from build123d import *

# Parameters (mm, degrees)
SKETCH1_R                = 67.8
SKETCH1_R_2              = 50
BOSS_EXTRUDE1_DEPTH      = 10
BOSS_EXTRUDE4_DEPTH      = 10
BOSS_EXTRUDE4_DEPTH_BACK = 10
SKETCH2_R                = 25
SKETCH2_R_2              = 67.8
CUT_EXTRUDE1_START       = -20
CUT_EXTRUDE1_DEPTH       = 20


# Read off the part's stored shape, not the designer's step: Cut-Extrude1
with BuildPart() as part:
    # Sketch1 → Boss-Extrude1 (new body)
    with BuildSketch(Plane(origin=(0, 0, 0), x_dir=(1, 0, 0), z_dir=(0, 1, 0))):
        with Locations(Location((0, 0, 0), (0, 0, 270))):
            Circle(SKETCH1_R)
        with Locations(Location((0, 0, 0), (0, 0, 270))):
            Circle(SKETCH1_R_2, mode=Mode.SUBTRACT)
    extrude(amount=BOSS_EXTRUDE1_DEPTH)

    # Sketch2 → Boss-Extrude4 (add, two sides: drawn at the far end of the back side and taken through both)
    with BuildSketch(Plane(origin=(0, 10, 0), x_dir=(1, 0, 0), z_dir=(0, 1, 0)).offset(-BOSS_EXTRUDE4_DEPTH_BACK)):
        with BuildLine():
            ThreePointArc((150, -40), (190, 0), (150, 40))
            ThreePointArc((150, 40), (134.692662705, 36.9551813), (121.715728753, 28.284271247))
            add(Edge.make_bspline(
                [(53.033008589, 53.033008589), (65.214190565, 40.851826613), (81.157405982, 26.386889755), (111.148754798, 17.717297293), (121.715728753, 28.284271247)],
                knots=[0, 0, 0, 0, 0.557862637, 1, 1, 1, 1], degree=3))
            ThreePointArc((53.033008589, 53.033008589), (0, 75), (-53.033008589, 53.033008589))
            add(Edge.make_bspline(
                [(-53.033008589, 53.033008589), (-65.214190565, 40.851826613), (-81.157405982, 26.386889755), (-111.148754798, 17.717297293), (-121.715728753, 28.284271247)],
                knots=[0, 0, 0, 0, 0.557862637, 1, 1, 1, 1], degree=3))
            ThreePointArc((-121.715728753, 28.284271247), (-134.692662705, 36.9551813), (-150, 40))
            ThreePointArc((-150, 40), (-190, 0), (-150, -40))
            ThreePointArc((-150, -40), (-134.692662705, -36.9551813), (-121.715728753, -28.284271247))
            add(Edge.make_bspline(
                [(-53.033008589, -53.033008589), (-65.214190565, -40.851826613), (-81.157405982, -26.386889755), (-111.148754798, -17.717297293), (-121.715728753, -28.284271247)],
                knots=[0, 0, 0, 0, 0.557862637, 1, 1, 1, 1], degree=3))
            ThreePointArc((-53.033008589, -53.033008589), (0, -75), (53.033008589, -53.033008589))
            add(Edge.make_bspline(
                [(53.033008589, -53.033008589), (65.214190565, -40.851826613), (81.157405982, -26.386889755), (111.148754798, -17.717297293), (121.715728753, -28.284271247)],
                knots=[0, 0, 0, 0, 0.557862637, 1, 1, 1, 1], degree=3))
            ThreePointArc((121.715728753, -28.284271247), (134.692662705, -36.9551813), (150, -40))
        make_face()
        with Locations(Location((-150, 0, 0), (0, 0, 270))):
            Circle(SKETCH2_R, mode=Mode.SUBTRACT)
        with Locations(Location((0, 0, 0), (0, 0, 270))):
            Circle(SKETCH2_R_2, mode=Mode.SUBTRACT)
        with Locations(Location((150, 0, 0), (0, 0, 270))):
            Circle(SKETCH2_R, mode=Mode.SUBTRACT)
    extrude(amount=BOSS_EXTRUDE4_DEPTH + BOSS_EXTRUDE4_DEPTH_BACK)

    # Cut-Extrude1 outline → Cut-Extrude1 (cut)
    with BuildSketch(Plane(origin=(0, 20, 0), x_dir=(1, 0, 0), z_dir=(0, 1, 0)).offset(CUT_EXTRUDE1_START)):
        with BuildLine():
            ThreePointArc((188.729833462, -10), (190, 0), (188.729833462, 10))
            Line((188.729833462, 10), (172.912878475, 10))
            ThreePointArc((172.912878475, 10), (175, 0), (172.912878475, -10))
            Line((172.912878475, -10), (188.729833462, -10))
        make_face()
        with BuildLine():
            ThreePointArc((-172.912878475, -10), (-175, 0), (-172.912878475, 10))
            Line((-172.912878475, 10), (-188.729833462, 10))
            ThreePointArc((-188.729833462, 10), (-190, 0), (-188.729833462, -10))
            Line((-188.729833462, -10), (-172.912878475, -10))
        make_face()
    extrude(amount=CUT_EXTRUDE1_DEPTH, mode=Mode.SUBTRACT)


solid = part.part
The model under review builds one solid part; all positions refer to its coordinate system, in mm. A direction names the side the tool comes from. Coordinates: 2 decimals unless noted, no trailing zeros. Loops run counter-clockwise (first coordinate to the right, second up) from the corner with the lowest first, then second, coordinate; pieces in that order, holes last.
(1) Tool access review of faces 5 (the cylindrical face through (15.02, 4.93, 47.69)), 6 (the flat face through (-50, 10, -5)), 7 (the flat face through (-181, 10, -10)), 8 (the flat face through (181, 10, 10)): name each direction out of +Z, -Z, +X, -X, +Y, -Y from which nothing blocks a thin tool from reaching the whole face with its end or side.
Determined:
face 5: +Y, -Y
face 6: +Y
face 7: -X, +Y, -Y
face 8: +X, +Y, -Y
(2) Consider section D-D, the plane z = 56.5. Give the boundary of the cut face in (x, y), plus the area to 3 significant figures.
Determined:
outline: (-49.32, 0) - (49.32, 0) - (49.32, 20) - (37.48, 20) - (37.48, 10) - (-37.48, 10) - (-37.48, 20) - (-49.32, 20) - close
area: 1,220 mm2
(3) Draft analysis for pull direction Z (two halves, no side actions). For faces 1 (the flat face through (13, 20, -67)), 2 (the cylindrical face through (-0.825, 9.86, 74.995)), 3 (the cylindrical face through (125.02, 9.86, -0.96)), 4 (the cylindrical face through (0.825, 9.86, -74.995)), state which applies: +Z half, -Z half, draft (parallel to the pull), parting line (faces both ways), or undercut.
Determined:
face 1: draft
face 2: +Z half
face 3: undercut
face 4: -Z half
(4) Insertion check: P1, Ø4, axis at y = 16, z = 59.5, coming from the +X side; P2, Ø5, axis at x = 105.5, y = 15.5, coming from the +Z side; P3, Ø2, axis at x = 38.5, z = -57, coming from the -Y side; P4, Ø6, axis at y = 8.5, z = 51, coming from the +X side. Each pin has a flat end and moves straight along its axis. Give the tip position at first contact, or say it passes through.
Determined:
P1: stops at x = 48.15
P2: stops at z = 21.68
P3: stops at y = 0
P4: stops at x = 58.13
(5) Consider section A-A, the plane z = 0. Give the boundary of the cut face in (x, y), plus the area to 3 significant figures.
Determined:
outline: (-125, 0) - (-50, 0) - (-50, 10) - (-67.8, 10) - (-67.8, 20) - (-125, 20) - close; (50, 0) - (125, 0) - (125, 20) - (67.8, 20) - (67.8, 10) - (50, 10) - close
area: 2,640 mm2
(6) Consider section B-B, the plane x = 0. Give the boundary of the cut face in (y, z), plus the area to 3 significant figures.
Determined:
outline: (0, -75) - (20, -75) - (20, -67.8) - (10, -67.8) - (10, -50) - (0, -50) - close; (0, 50) - (10, 50) - (10, 67.8) - (20, 67.8) - (20, 75) - (0, 75) - close
area: 644 mm2
(7) Wall thickness on L1, parallel to X at y = 5.5, z = 0; L2, parallel to X at y = 15, z = 1; L3, parallel to X at y = 1.5, z = 15: over which ranges is each line inside the solid? List them lowest first.
Determined:
L1: x = -125 to -50, 50 to 125
L2: x = -125.02 to -67.79, 67.79 to 125.02
L3: x = -187.08 to -170, -130 to -47.7, 47.7 to 130, 170 to 187.08
(8) Consider section C-C, the plane x = -134.5. Give the boundary of the cut face in (y, z), plus the area to 3 significant figures.
Determined:
outline: (0, -36.87) - (20, -36.87) - (20, -19.62) - (0, -19.62) - close; (0, 19.62) - (20, 19.62) - (20, 36.87) - (0, 36.87) - close
area: 690 mm2
